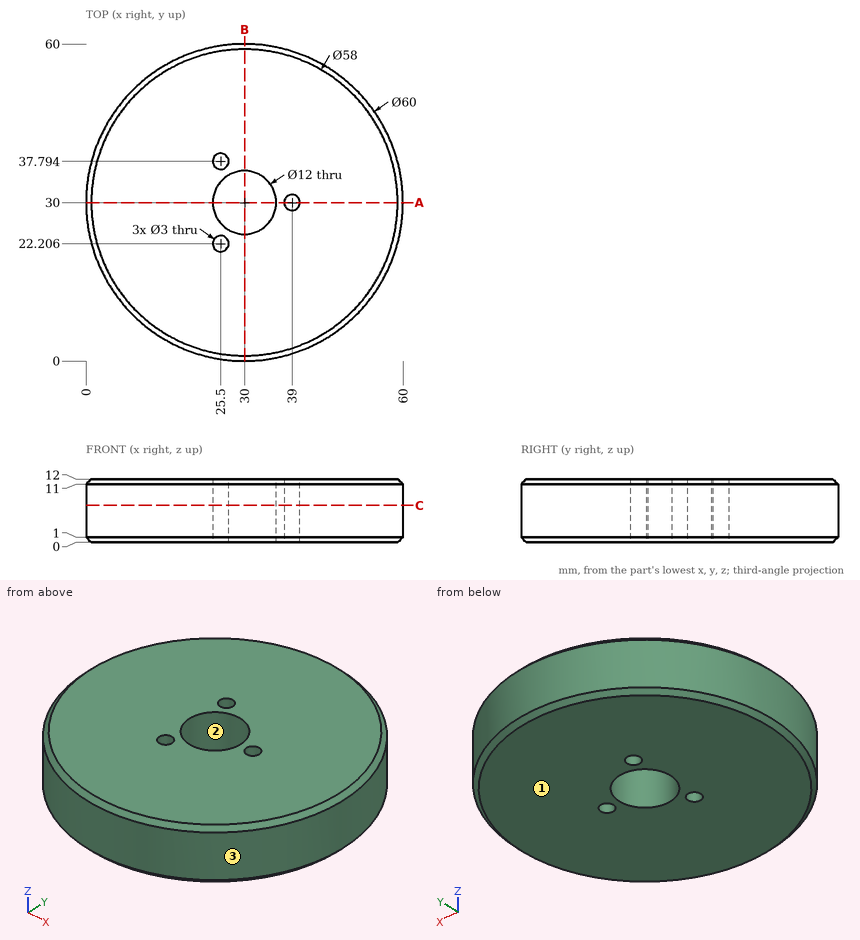
Drawing for the job (mm, zero at the part's lowest x, y, z). Give positions to 0.01 mm unless a question says otherwise; leave off trailing zeros. Write each loop counter-clockwise with the first axis right and the second up, starting at its lowest first coordinate (ties: lowest second). Pieces come first, ordered by that corner, then holes. Notation, with made-up numbers: M 25,7.25 L 71,7.25 A29 cw 71,31.25 Z; hole C 25.5,30 d11. An arc over 180 degrees is marked long. Return JSON: item names as keys, results as strings. Group by question number.
(1) Drill centre lines: L1, parallel to Y at x = 30, z = 9; L2, parallel to Y at x = 25.5, z = 6.25 (1 decimal); L3, parallel to Y at x = 39, z = 5.75. Where is each one in solid material? Low to high. Write a range as [from, to].
(2) Band-saw the part on C-C (z = 7). Give the cut face in (x, y).
(3) Band-saw the part on B-B (x = 30). Give the cut face in (y, z), and give its area (3 significant figures).
(4) Flat gauge pins, fed straight in: pin 1 Ø9.5 at (x, y) = (30, 30) entering from -Z; pin 2 Ø5 at (x, y) = (21.5, 43.5) entering from -Z; pin 3 Ø2 at (x, z) = (41, 8.5) entering from +Y; pin 4 Ø5 at (x, z) = (42, 7.5) entering from -Y. Where does each tip first touch, or does it go through?
(5) Band-saw the part on A-A (y = 30). Give the cut face in (x, z), and give its area (3 significant figures).
(6) Mould opens along X. For the marked faces 1, 2 and 3 say: pulls with the +X half, pulls with the -X half, needs draft (parallel to the pull), parting line crosses it, or undercut.
Entries:
{
 "1": {"L1": "y = [0, 24], [36, 60]", "L2": "y = [0.3, 20.7], [23.7, 26], [34, 36.3], [39.3, 59.7]", "L3": "y = [1.38, 28.5], [31.5, 58.62]"},
 "2": {"outline": "C 30,30 d60; hole C 25.5,22.21 d3; hole C 30,30 d12; hole C 25.5,37.79 d3; hole C 39,30 d3"},
 "3": {"outline": "M 0,1 L 1,0 L 24,0 L 24,12 L 1,12 L 0,11 Z; M 36,0 L 59,0 L 60,1 L 60,11 L 59,12 L 36,12 Z", "area": "574 mm^2"},
 "4": {"pin 1": "passes through", "pin 2": "stops at z = 0", "pin 3": "stops at y = 58.28", "pin 4": "stops at y = 1.54"},
 "5": {"outline": "M 0,1 L 1,0 L 24,0 L 24,12 L 1,12 L 0,11 Z; M 36,0 L 37.5,0 L 37.5,12 L 36,12 Z; M 40.5,0 L 59,0 L 60,1 L 60,11 L 59,12 L 40.5,12 Z", "area": "538 mm^2"},
 "6": {"face 1": "needs draft", "face 2": "undercut", "face 3": "parting line crosses it"}
}
